Verification items for the finished model (mm, model axes). Round coordinates to 2 decimals unless told otherwise and drop trailing zeros. Write each loop counter-clockwise with the first axis right and the second up, starting at its lowest first coordinate (ties: lowest second). Pieces come first, ordered by that corner, then holes. Notation, with made-up numbers: M -5,12 L 0,12 A9 cw 0,27 Z; hole C 74,13 d9. An arc over 180 degrees is marked long. One line per question, with ' | ' between items. Start each with the question number.
Q1. Cross-section at B-B (x = 637). Record the boundary of the cut face in (y, z), then the cut area to 3 significant figures.
Q2. Gauge pin test, flat ends, axial feed: pin 1 (3 mm diameter, centred on x = 699.5, z = 0, fed in from -Y); pin 2 (5 mm diameter, centred on x = 153.5, z = -3.5, fed in from -Y); pin 3 (2 mm diameter, centred on x = 325, y = -2.5, fed in from -Z); pin 4 (4 mm diameter, centred on x = 11.5, y = -2.5, fed in from +Z). Record the tip position at first contact, or that the pin passes through.
Q3. Cross-section at A-A (y = 0). Record the boundary of the cut face in (x, z), then the cut area to 3 significant figures.
Q4. Thickness scan on line 1 along X through (y, z) = (3.25, 0); line 2 along Z through (x, y) = (699.5, 4); line 3 along X through (y, z) = (-3.5, 0). Record the ranges inside material, lowest first. Write a range as from..to.
from build123d import *

# Parameters (mm, degrees)
SKETCH_1_R               = 8
EXTRUDE_1_DEPTH          = 703.5
SKETCH_2_R               = 4
CUT_EXTRUDE_1_DEPTH      = 9
CUT_EXTRUDE_1_DEPTH_BACK = 9
SKETCH_3_OUTSIDE_W       = 158.772
SKETCH_3_OUTSIDE_H       = 158.772
SKETCH_3_OUTSIDE_W_2     = 8
SKETCH_3_OUTSIDE_H_2     = 20
CUT_EXTRUDE_2_DEPTH      = 20
SKETCH_4_R               = 2
CUT_EXTRUDE_3_DEPTH      = 25


with BuildPart() as part:
    # 草图1 → 凸台-拉伸1 (new body)
    with BuildSketch(Plane(origin=(0, 0, 0), x_dir=(0, 0, -1), z_dir=(1, 0, 0))):
        Circle(SKETCH_1_R)
    extrude(amount=EXTRUDE_1_DEPTH)

    # 草图2 → 切除-拉伸1 (cut, two sides)
    with BuildSketch(Plane.XY) as cut_extrude_1_sk:
        with Locations((10, 0)):
            Circle(SKETCH_2_R)
    extrude(amount=CUT_EXTRUDE_1_DEPTH, mode=Mode.SUBTRACT)
    extrude(cut_extrude_1_sk.sketch, amount=-CUT_EXTRUDE_1_DEPTH_BACK, mode=Mode.SUBTRACT)

    # 草图3 outside → 切除-拉伸2 (cut)
    with BuildSketch(Plane.ZY):
        Rectangle(SKETCH_3_OUTSIDE_W, SKETCH_3_OUTSIDE_H)
        Rectangle(SKETCH_3_OUTSIDE_W_2, SKETCH_3_OUTSIDE_H_2, mode=Mode.SUBTRACT)
    extrude(amount=-CUT_EXTRUDE_2_DEPTH, mode=Mode.SUBTRACT)

    # 草图4 → 切除-拉伸3 (cut, symmetric)
    with BuildSketch(Plane(origin=(0, 0, 0), x_dir=(1, 0, 0), z_dir=(0, 1, 0))):
        with Locations((699.5, 0)):
            Circle(SKETCH_4_R)
    extrude(amount=CUT_EXTRUDE_3_DEPTH, both=True, mode=Mode.SUBTRACT)


solid = part.part
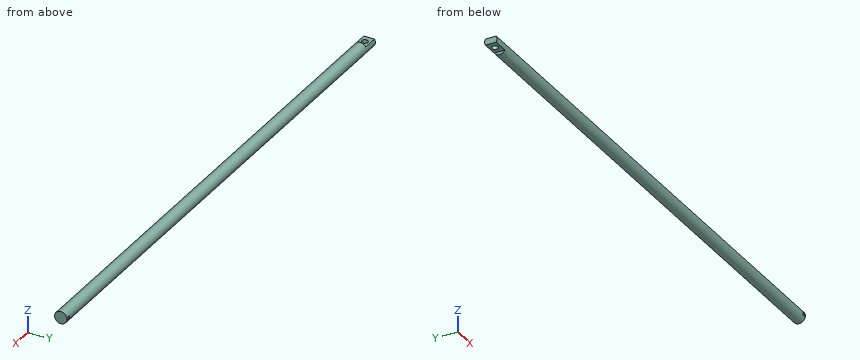
Determined:
1) outline: C 0,0 d16 | area: 201 mm²
2) pin 1: passes through | pin 2: stops at y = -7.94 | pin 3: stops at z = -7.86 | pin 4: stops at z = 4
3) outline: M 0,-4 L 6,-4 L 6,4 L 0,4 Z; M 14,-4 L 20,-4 L 20,-8 L 703.5,-8 L 703.5,8 L 20,8 L 20,4 L 14,4 Z; hole C 699.5,0 d4 | area: 11,000 mm²
4) line 1: x = 0..7.67, 12.33..697.5, 701.5..703.5 | line 2: z = -6.93..-2, 2..6.93 | line 3: x = 0..8.06, 11.94..697.5, 701.5..703.5
